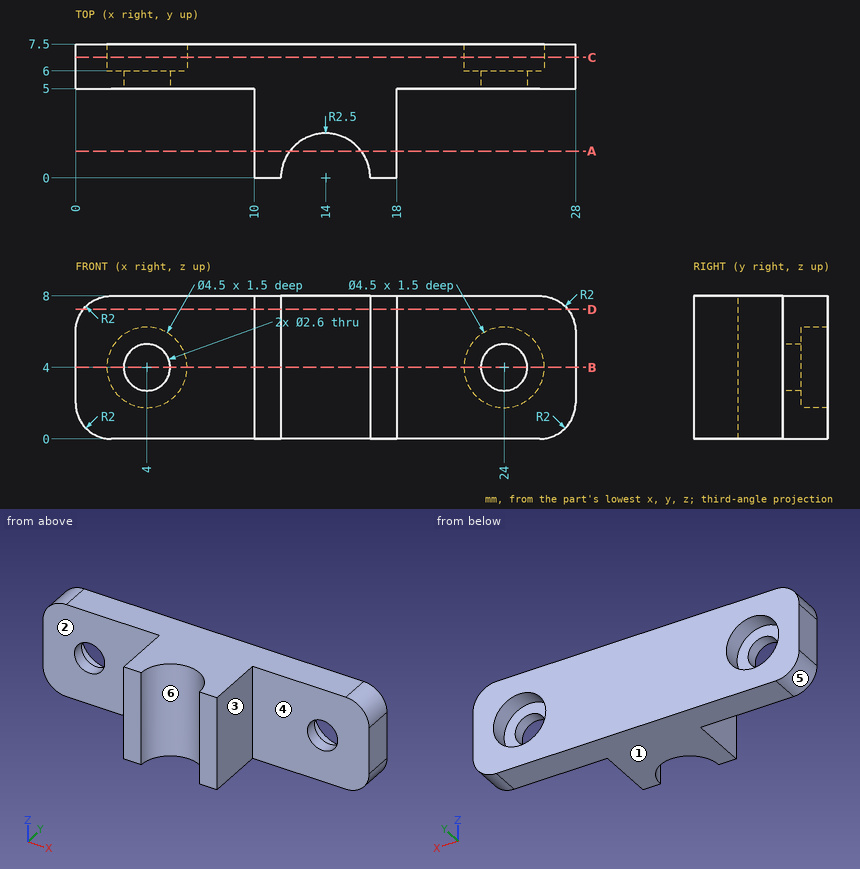
Could you check a few things on this drawing? It's one solid part, dimensions in mm from its lowest x, y, z. A direction names the side the tool comes from. Coordinates: 2 decimals unless noted, no trailing zeros. Order: outer loops, then holes, each group sorted by start corner. A loop starts at its lowest first (then second) coordinate and runs counter-clockwise, first axis right, second up. Notation, with made-up numbers: M -31.5,44 L 12.5,44 A13 ccw 12.5,55 Z; hole C -25.75,4.5 d11. An arc over 180 degrees is marked long. Use one line per item in the form item = value. Start each with the question number.
1. Please list where these lines run through material, in increasing order: line 1 (Z direction, x = 4, y = 7.1); line 2 (Z direction, x = 4, y = 5.3); line 3 (Y direction, x = 21.5, z = 4.25).
2. We'd pull the mould along X, two halves only. Please class the marked faces 4, 5 and 6: +X half, -X half, draft (parallel to the pull), parting line (faces both ways), or undercut.
3. For pin 1 (3 mm diameter, centred on x = 4, z = 4, fed in from -Y); pin 2 (3.5 mm diameter, centred on x = 24, z = 4, fed in from +Y); pin 3 (2.5 mm diameter, centred on y = 2, z = 4.5, fed in from +X), each with a flat end and sliding along its axis, tell me the tip position at first contact or that it passes through.
4. Suppose I cut it at A-A on y = 1.5. Write out the boundary of the cut face in (x, z).
5. Suppose I cut it at C-C on y = 6.75. Write out the boundary of the cut face in (x, z), then the cut area to 3 significant figures.
6. Suppose I cut it at D-D on z = 7.25. Write out the boundary of the cut face in (x, y), then the cut area to 3 significant figures.
7. On a 3-axis mill with a long thin cutter (end or side, diameter ignored), from which of +Z, -Z, +X, -X, +Y, -Y can I reach the whole of each face in a straight line? I mean the marked faces 1, 2 and 3. Say none if no direction works.
8. Suppose I cut it at B-B on z = 4. Write out the boundary of the cut face in (x, y).
Geometry says:
q1.line_1 = 0 to 1.75, 6.25 to 8
q1.line_2 = 0 to 2.7, 5.3 to 8
q1.line_3 = 5 to 7.5
q2.face_4 = draft
q2.face_5 = -X half
q2.face_6 = undercut
q3.pin_1 = 5
q3.pin_2 = 6
q3.pin_3 = 18
q4.outline = M 10,0 L 12,0 L 12,8 L 10,8 Z; M 16,0 L 18,0 L 18,8 L 16,8 Z
q5.outline = M 0,2 A2 ccw 2,0 L 26,0 A2 ccw 28,2 L 28,6 A2 ccw 26,8 L 2,8 A2 ccw 0,6 Z; hole C 4,4 d4.5; hole C 24,4 d4.5
q5.area = 189 mm^2
q6.outline = M 0.44,5 L 10,5 L 10,0 L 11.5,0 A2.5 cw 16.5,0 L 18,0 L 18,5 L 27.56,5 L 27.56,7.5 L 0.44,7.5 Z
q6.area = 98.0 mm^2
q7.face_1 = -Z, +X, -X, +Y, -Y
q7.face_2 = +Z, -Z, -X, -Y
q7.face_3 = +Z, -Z, +X, -Y
q8.outline = M 0,5 L 2.7,5 L 2.7,6 L 1.75,6 L 1.75,7.5 L 0,7.5 Z; M 5.3,5 L 10,5 L 10,0 L 11.5,0 A2.5 cw 16.5,0 L 18,0 L 18,5 L 22.7,5 L 22.7,6 L 21.75,6 L 21.75,7.5 L 6.25,7.5 L 6.25,6 L 5.3,6 Z; M 25.3,5 L 28,5 L 28,7.5 L 26.25,7.5 L 26.25,6 L 25.3,6 Z
